```python
from build123d import *

# Parameters (mm, degrees)
PAD017_DEPTH           = 5
PAD020_DEPTH           = 6.25
SKETCH059_W            = 7.7
SKETCH059_H            = 1.65
PAD029_DEPTH           = 7.5
SKETCH056_W            = 7.7
SKETCH056_H            = 1.65
PAD030_DEPTH           = 4.6
SKETCH058_W            = 7.7
SKETCH058_H            = 1.65
PAD031_DEPTH           = 7.5
SKETCH057_W            = 4.6
SKETCH057_H            = 1.65
PAD032_DEPTH           = 7.5
LINEARPATTERN012_COUNT = 2
LINEARPATTERN012_PITCH = 3.3
CHAMFER002_SIZE        = 1


with BuildPart() as obj1:
    # Sketch034 → Pad017 (new body)
    with BuildSketch(Plane.XY):
        with BuildLine():
            Line((-1.35, -1.8), (-1.35, 6))
            ThreePointArc((0, 7.35), (-0.954594, 6.954594), (-1.35, 6))
            Line((0, 9), (0, 7.35))
            Line((-2.6, 9), (0, 9))
            Line((-2.6, -1.8), (-2.6, 9))
            Line((-3.85, -1.8), (-2.6, -1.8))
            ThreePointArc((-3.85, -1.8), (-3.439949, -2.789949), (-2.45, -3.2))
            Line((-1.35, -3.2), (-2.45, -3.2))
            Line((-1.35, -1.8), (-1.35, -3.2))
        make_face()
    extrude(amount=PAD017_DEPTH)

    # Sketch037 → Pad020 (join)
    with BuildSketch(Plane.XY):
        Polygon((-1.35, 0.2), (-1.35, 1.6), (-2.6, 1.6), (-3.85, 1.6), (-3, 0.2), (-2.6, 0.2), align=None)
    extrude(amount=PAD020_DEPTH)


with BuildPart() as obj2:
    # Mirror001: instance of _obj1
    add(obj1.part.mirror(Plane(origin=(0, 0, 0), x_dir=(0, 1, 0), z_dir=(-1, 0, 0))))


with BuildPart() as body015:
    # Fusion001 base: copy of _obj1
    add(obj1.part)

    # Fusion001: union _obj2)
    add(obj2.part)

    # Sketch059 → Pad029 (new body)
    with BuildSketch(Plane.XY):
        with Locations((-1.25, 8.175)):
            Rectangle(SKETCH059_W, SKETCH059_H)
    extrude(amount=PAD029_DEPTH)

    # Sketch056 → Pad030 (join)
    with BuildSketch(Plane.XY):
        with Locations((-1.25, 9.825)):
            Rectangle(SKETCH056_W, SKETCH056_H)
    pad030 = extrude(amount=PAD030_DEPTH)

    # Sketch058 → Pad031 (join)
    with BuildSketch(Plane.XY):
        with Locations((-1.25, 11.475)):
            Rectangle(SKETCH058_W, SKETCH058_H)
    pad031 = extrude(amount=PAD031_DEPTH)

    # Sketch057 → Pad032 (join)
    with BuildSketch(Plane.XY):
        with Locations((0.3, 9.825)):
            Rectangle(SKETCH057_W, SKETCH057_H)
    pad032 = extrude(amount=PAD032_DEPTH)

    # LinearPattern012: Pad030, Pad031, Pad032 ×2
    with Locations(*[(0, i * LINEARPATTERN012_PITCH, 0) for i in range(1, LINEARPATTERN012_COUNT)]):
        add(pad030)
        add(pad031)
        add(pad032)

    # Chamfer002
    chamfer002_edges = [body015.edges().sort_by_distance(p)[0] for p in [
        (-5.1, 14.775, 7.5),
        (-5.1, 11.475, 7.5),
        (-5.1, 8.175, 7.5),
    ]]
    chamfer(chamfer002_edges, length=CHAMFER002_SIZE)


solid = body015.part
```
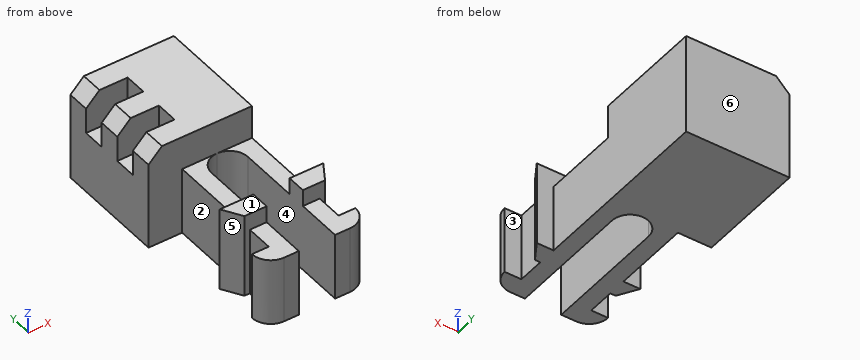
Geometry check sheet. Reference: the model listing, model coordinates, mm. Face numbers are marked on the shaded views. A direction names the side the tool comes from. Round coordinates to 2 decimals unless told otherwise and drop trailing zeros. Order: outer loops, then holes, each group sorted by start corner. A loop starts at its lowest first (then second) coordinate and runs counter-clockwise, first axis right, second up. Notation, with made-up numbers: (3.25, -28) -> (22.25, -28) arc R8 cw to (22.25, -13) -> close; hole circle Ø4 at (58, 13.5). An arc over 180 degrees is marked (long way). Return JSON: item names as keys, results as strings. Group by question number.
Q1. Section check C-C, the plane z = 1.25. Record the boundary of the cut face in (x, y).
Q2. Section check B-B, the plane x = -2.25. Record the boundary of the cut face in (y, z), plus the area to 3 significant figures.
Q3. Material ranges on probe 1 along Y at (x, z) = (-2.25, 7); probe 2 along Y at (x, z) = (-2.75, 2.75); probe 3 along X at (y, z) = (3.5, 2.5), recorded low to high. Write a range as from..to.
Q4. Section check A-A, the plane y = 1. Record the boundary of the cut face in (x, z).
Q5. Release check for a two-part mould opening along X. For the marked faces 4, 5 and 6 record: released by +X, released by -X, zero draft, split by the parting line, or undercut.
Q6. Section check D-D, the plane x = -3.5. Record the boundary of the cut face in (y, z).
Q7. Gauge pin test, flat ends, axial feed: pin 1 (0.8 mm diameter, centred on x = 1, y = 5.5, fed in from +Z); pin 2 (0.9 mm diameter, centred on x = -4, z = 6, fed in from -Y); pin 3 (2 mm diameter, centred on y = 10, z = 3.5, fed in from +X). Record the tip position at first contact, or that the pin passes through.
Q8. Tool access check on the marked faces 1, 2 and 3. Record the directions out of +Z, -Z, +X, -X, +Y, -Y that give a thin tool (end or side, any length) a straight path to the whole face; none if there is none.
Numbers:
{
 "1": {"outline": "(-5.1, 7.35) -> (-2.6, 7.35) -> (-2.6, 1.6) -> (-3.85, 1.6) -> (-3, 0.2) -> (-2.6, 0.2) -> (-2.6, -1.8) -> (-3.85, -1.8) arc R1.4 ccw to (-2.45, -3.2) -> (-1.35, -3.2) -> (-1.35, 6) arc R1.35 cw to (0, 7.35) arc R1.35 cw to (1.35, 6) -> (1.35, -3.2) -> (2.45, -3.2) arc R1.4 ccw to (3.85, -1.8) -> (2.6, -1.8) -> (2.6, 0.2) -> (3, 0.2) -> (3.85, 1.6) -> (2.6, 1.6) -> (2.6, 15.6) -> (-5.1, 15.6) -> close"},
 "2": {"outline": "(-3.2, 0) -> (15.6, 0) -> (15.6, 7.5) -> (13.95, 7.5) -> (13.95, 4.6) -> (12.3, 4.6) -> (12.3, 7.5) -> (10.65, 7.5) -> (10.65, 4.6) -> (9, 4.6) -> (9, 7.5) -> (7.35, 7.5) -> (7.35, 5) -> (1.6, 5) -> (1.6, 6.25) -> (0.2, 6.25) -> (0.2, 5) -> (-3.2, 5) -> close", "area": "107 mm^2"},
 "3": {"probe 1": "7.35..9, 10.65..12.3, 13.95..15.6", "probe 2": "-3.17..-1.8, 0.2..1.6, 7.35..15.6", "probe 3": "-2.6..-1.35, 1.35..2.6"},
 "4": {"outline": "(-3.49, 0) -> (-1.35, 0) -> (-1.35, 6.25) -> (-3.49, 6.25) -> close; (1.35, 0) -> (3.49, 0) -> (3.49, 6.25) -> (1.35, 6.25) -> close"},
 "5": {"face 4": "undercut", "face 5": "released by -X", "face 6": "zero draft"},
 "6": {"outline": "(-2.73, 0) -> (-1.8, 0) -> (-1.8, 5) -> (-2.73, 5) -> close; (1.02, 0) -> (1.6, 0) -> (1.6, 6.25) -> (1.02, 6.25) -> close; (7.35, 0) -> (15.6, 0) -> (15.6, 7.5) -> (13.95, 7.5) -> (13.95, 4.6) -> (12.3, 4.6) -> (12.3, 7.5) -> (10.65, 7.5) -> (10.65, 4.6) -> (9, 4.6) -> (9, 7.5) -> (7.35, 7.5) -> close"},
 "7": {"pin 1": "z = 5", "pin 2": "y = 1.11", "pin 3": "x = 2.6"},
 "8": {"face 1": "+Z, +X, -X, -Y", "face 2": "+Z, -Z, -X", "face 3": "+Z, -Z, +X"}
}
